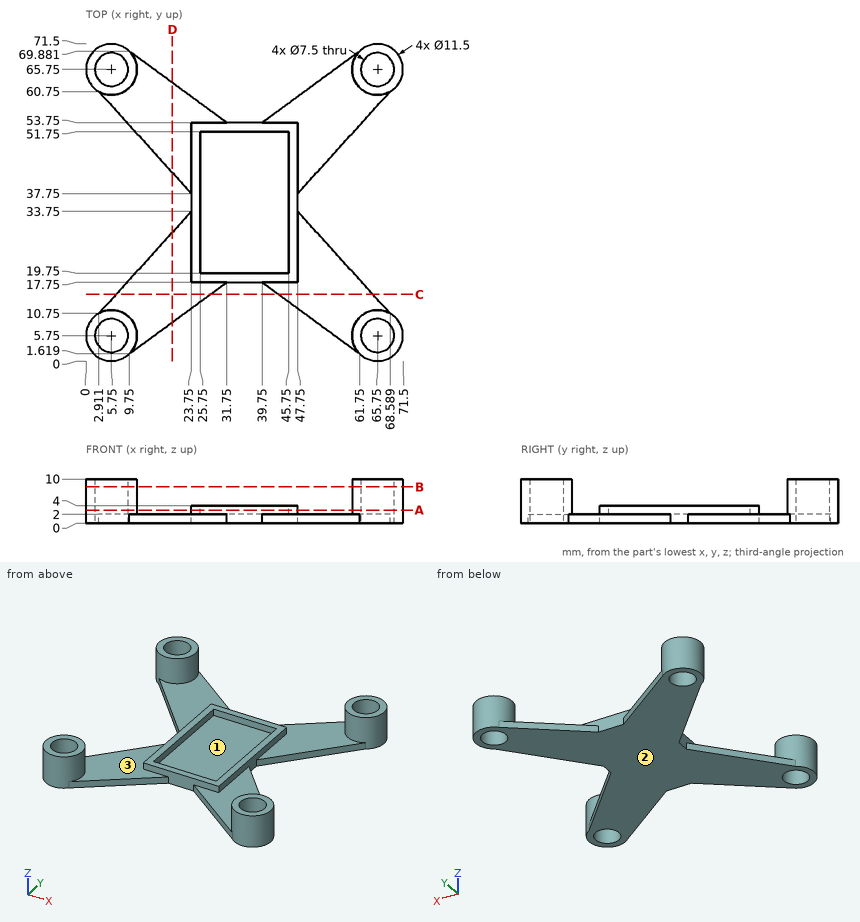
Source: three-view drawing plus pictorial views. Frame: mm from the lowest corner of the part. Round coordinates to 2 decimals unless told otherwise and drop trailing zeros. Loops run counter-clockwise (first coordinate to the right, second up) from the corner with the lowest first, then second, coordinate; pieces in that order, holes last.
Q1. Section D-D, the plane x = 19.5. Return loops of the section in (y, z).
Q2. Section C-C, the plane y = 15. Return loops of the section in (x, z).
Q3. First-contact query: P1, Ø2, axis at y = 41, z = 4, coming from the -X side; P2, Ø4.5, axis at x = 32.5, z = 1, coming from the -Y side; P3, Ø12, axis at x = 36, y = 27, coming from the +Z side; P4, Ø4, axis at y = 57.5, z = 5, coming from the +X side. Flat tips, straight axial feed; report the tip coordinate or a pass-through.
Q4. Section B-B, the plane z = 8.25. Return loops of the section in (x, y), plus the area to 3 significant figures.
Q5. Mould query, pull axis X, two halves, no side actions, for the marked faces 1, 2 and 3. Classes: pulls with the +X half, pulls with the -X half, needs draft (parallel to the pull), parting line crosses it, or undercut.
Q6. Section A-A, the plane z = 3. State how many separate pieces and enclosed holes the cut face has.
Q7. Ray query, line 1 (X direction, y = 65.75, z = 2.25); line 2 (Y direction, x = 64, z = 4) (1 decimal). Return the intervals inside material, ascending.
Solutions:
1. outline: (8.77, 0) - (29.06, 0) - (29.06, 2) - (8.77, 2) - close; (42.44, 0) - (62.73, 0) - (62.73, 2) - (42.44, 2) - close
2. outline: (6.76, 0) - (28, 0) - (28, 2) - (6.76, 2) - close; (43.5, 0) - (64.74, 0) - (64.74, 2) - (43.5, 2) - close
3. P1: stops at x = 23.75
3. P2: stops at y = 16.65
3. P3: stops at z = 2
3. P4: passes through
4. outline: circle Ø11.5 at (5.75, 5.75); circle Ø11.5 at (5.75, 65.75); circle Ø11.5 at (65.75, 5.75); circle Ø11.5 at (65.75, 65.75); hole circle Ø7.5 at (5.75, 5.75); hole circle Ø7.5 at (5.75, 65.75); hole circle Ø7.5 at (65.75, 5.75); hole circle Ø7.5 at (65.75, 65.75)
4. area: 239 mm2
5. face 1: undercut
5. face 2: needs draft
5. face 3: undercut
6. separate pieces: 5
6. enclosed holes: 5
7. line 1: x = 0 to 2, 9.5 to 11.5, 60 to 62, 69.5 to 71.5
7. line 2: y = 0.3 to 2.4, 9.1 to 11.2, 60.3 to 62.4, 69.1 to 71.2
